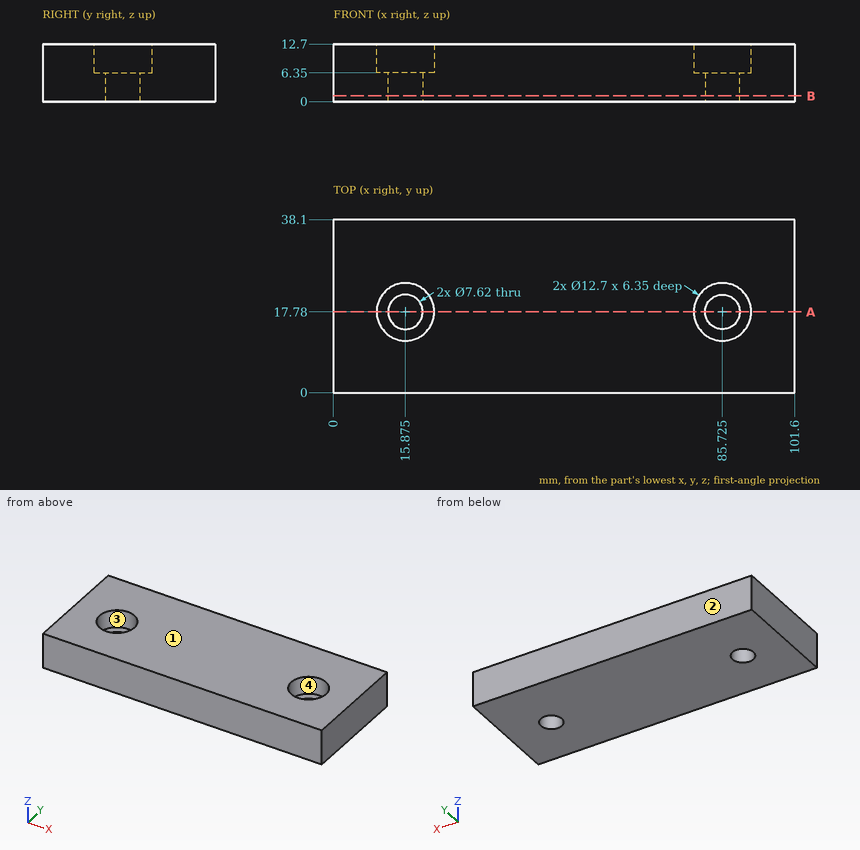
Part print with two shaded views. Sizes in mm from the minimum x, y, z corner. Coordinates: 2 decimals unless noted, no trailing zeros. Write each loop counter-clockwise with the first axis right and the second up, starting at its lowest first coordinate (ties: lowest second). Pieces come first, ordered by that corner, then holes.
(1) Pin check, flat tip, straight feed: pin 1 Ø14 at (x, y) = (15.5, 15.5) entering from +Z. Stop position of the tip, or through.
(2) Cut at A-A on y = 17.78. List the corners of the cut face in (x, z) (3 decimals), and give its area (3 significant figures).
(3) Mould opens along Y. For the marked faces 1, 2, 3 and 4 say: pulls with the +Y half, pulls with the -Y half, needs draft (parallel to the pull), parting line crosses it, or undercut.
(4) Cut at B-B on z = 1.25. List the corners of the cut face in (x, y) (3 decimals), and give its area (3 significant figures).
(5) Drill centre lines: line 1 (X direction, y = 15, z = 2.5); line 2 (Y direction, x = 13, z = 12.25); line 3 (X direction, y = 14.5, z = 8.5). Where is each one in solid material? Low to high.
Working result:
1. pin 1: stops at z = 12.7
2. outline: (0, 0) - (12.065, 0) - (12.065, 6.35) - (9.525, 6.35) - (9.525, 12.7) - (0, 12.7) - close; (19.685, 0) - (81.915, 0) - (81.915, 6.35) - (79.375, 6.35) - (79.375, 12.7) - (22.225, 12.7) - (22.225, 6.35) - (19.685, 6.35) - close; (89.535, 0) - (101.6, 0) - (101.6, 12.7) - (92.075, 12.7) - (92.075, 6.35) - (89.535, 6.35) - close
2. area: 1,030 mm2
3. face 1: needs draft
3. face 2: pulls with the +Y half
3. face 3: undercut
3. face 4: undercut
4. outline: (0, 0) - (101.6, 0) - (101.6, 38.1) - (0, 38.1) - close; hole circle Ø7.62 at (15.875, 17.78); hole circle Ø7.62 at (85.725, 17.78)
4. area: 3,780 mm2
5. line 1: x = 0 to 13.27, 18.48 to 83.12, 88.33 to 101.6
5. line 2: y = 0 to 12.12, 23.44 to 38.1
5. line 3: x = 0 to 10.44, 21.31 to 80.29, 91.16 to 101.6
